Source: three-view drawing plus pictorial views. Frame: mm from the lowest corner of the part. A direction names the side the tool comes from. Round coordinates to 2 decimals unless told otherwise and drop trailing zeros. Loops run counter-clockwise (first coordinate to the right, second up) from the corner with the lowest first, then second, coordinate; pieces in that order, holes last. Notation, with made-up numbers: M 61,59.5 L 117,59.5 A18 cw 117,84.5 Z; hole C 31,23.5 d7. An arc over 180 degrees is marked long. Answer as a JSON object with one key per item and string values.
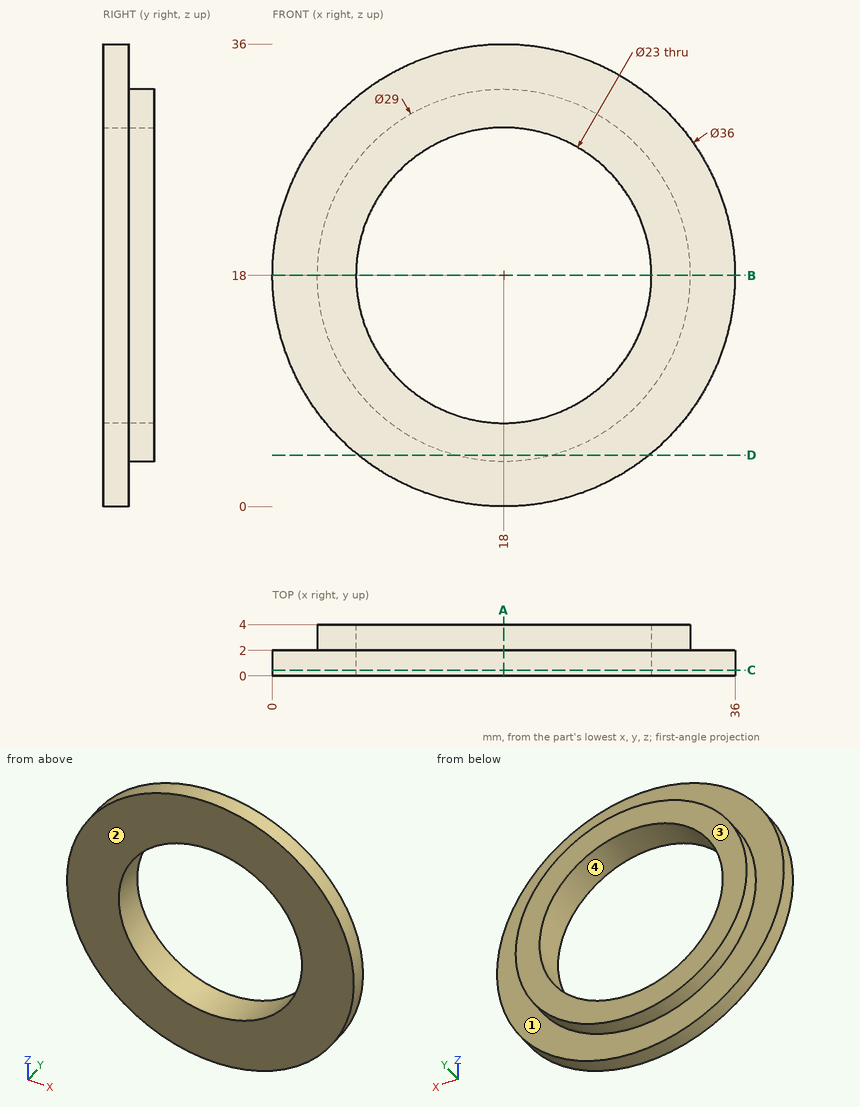
1) Cut plane A-A on x = 18. Return the cut outline in (y, z).
Geometry results:
{"outline": "M 0,0 L 2,0 L 2,3.5 L 4,3.5 L 4,6.5 L 0,6.5 Z; M 0,29.5 L 4,29.5 L 4,32.5 L 2,32.5 L 2,36 L 0,36 Z"}
2) Pull-direction query (Z, two-part tool) for the marked faces 3 and 4; classes: +Z half, -Z half, draft (parallel to the pull), parting line (faces both ways), or undercut.
Geometry results:
{"face 3": "draft", "face 4": "undercut"}
3) Set-up query: the marked faces 1 and 2. Return all of +Z, -Z, +X, -X, +Y, -Y with unobstructed straight access to the full face (end or side cutting, diameter ignored); none if empty.
Geometry results:
{"face 1": "+Y", "face 2": "+Z, -Z, +X, -X, -Y"}
4) Cut plane D-D on z = 4. Return the cut outline in (x, y).
Geometry results:
{"outline": "M 6.69,0 L 29.31,0 L 29.31,2 L 21.77,2 L 21.77,4 L 14.23,4 L 14.23,2 L 6.69,2 Z"}
5) First-contact query: pin 1 (3 mm diameter, centred on x = 11.5, z = 12.5, fed in from -Y); pin 2 (1.5 mm diameter, centred on y = 2.5, z = 11.5, fed in from +X). Flat tips, straight axial feed; report the tip coordinate or a pass-through.
Geometry results:
{"pin 1": "through", "pin 2": "x = 34.99"}
6) Cut plane B-B on z = 18. Return the cut outline in (x, y), and give its area (3 significant figures).
Geometry results:
{"outline": "M 0,0 L 6.5,0 L 6.5,4 L 3.5,4 L 3.5,2 L 0,2 Z; M 29.5,0 L 36,0 L 36,2 L 32.5,2 L 32.5,4 L 29.5,4 Z", "area": "38.0 mm2"}
7) Line query: probe 1 along X at (y, z) = (2.4, 18); probe 2 along X at (y, z) = (0.4, 18.5); probe 3 along Z at (x, y) = (15, 2.15). Output: solid intervals per line, ascending.
Geometry results:
{"probe 1": "3.5 to 6.5, 29.5 to 32.5", "probe 2": "0.01 to 6.51, 29.49 to 35.99", "probe 3": "3.81 to 6.9, 29.1 to 32.19"}
8) Cut plane C-C on y = 0.45. Return the cut outline in (x, z).
Geometry results:
{"outline": "C 18,18 d36; hole C 18,18 d23"}
